The listing builds one solid part. Answer for the finished solid, in the listing's coordinates (mm). Round coordinates to 2 decimals unless told otherwise and drop trailing zeros. Order: outer loops, then holes, each group sorted by start corner. A loop starts at its lowest first (then second) coordinate and runs counter-clockwise, first axis right, second up. Notation, with made-up numbers: (15.25, 56) -> (64.25, 56) arc R20 cw to (64.25, 62) -> close; hole circle Ø10 at (53, 80). An arc over 180 degrees is marked (long way). Answer in a Markdown table with one row per item. Add a question column.
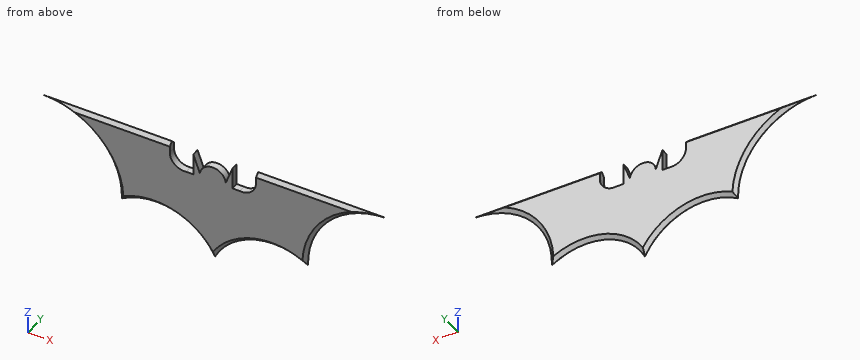
```python
from build123d import *

# Parameters (mm, degrees)
F1_DEPTH = 1.27
F2_SIZE  = 1.26999


# Not quite as in the source:
# - a fillet or chamfer is up to 0.001 mm smaller than in the source, because OpenCascade refuses the exact size
# - a feature names something its author has since deleted; it is built from what else it names


with BuildPart() as f1:
    # F0 (on Front) → F1 (new body, symmetric)
    with BuildSketch(Plane.XZ):
        with BuildLine():
            Line((-15.113, 14.986), (-60.325, 14.986))
            ThreePointArc((-60.325, 14.986), (-40.4178225843, 6.541072822), (-32.6550259817, -13.6418778197))
            ThreePointArc((-32.6550259817, -13.6418778197), (-14.2166113122, -11.1006310534), (0, -23.114))
            ThreePointArc((0, -23.114), (14.2166113122, -11.1006310534), (32.6550259817, -13.6418778197))
            ThreePointArc((32.6550259817, -13.6418778197), (40.4178225843, 6.541072822), (60.325, 14.986))
            Line((60.325, 14.986), (15.113, 14.986))
            Line((15.113, 14.986), (15.113, 11.43))
            ThreePointArc((15.113, 11.43), (13.3972241951, 7.623637489), (9.4089072578, 6.3884815532))
            Line((9.4089072578, 6.3884815532), (6.8689072578, 6.3884815532))
            Line((6.8689072578, 6.3884815532), (6.8689072578, 14.0084815532))
            Line((6.8689072578, 14.0084815532), (4.5436901303, 7.62))
            ThreePointArc((4.5436901303, 7.62), (0, 11.684), (-4.5436901303, 7.62))
            Line((-4.5436901303, 7.62), (-6.8689072578, 14.0084815532))
            Line((-6.8689072578, 14.0084815532), (-6.8689072578, 6.3884815532))
            Line((-6.8689072578, 6.3884815532), (-9.4089072578, 6.3884815532))
            ThreePointArc((-9.4089072578, 6.3884815532), (-13.3972241951, 7.623637489), (-15.113, 11.43))
            Line((-15.113, 11.43), (-15.113, 14.986))
        make_face()
    extrude(amount=F1_DEPTH, both=True)

    # F2 (size 1.27 in the source; OpenCascade refuses exactly that, so slightly less here)
    f2_edges = [f1.edges().sort_by_distance(p)[0] for p in [
        (-40.417823, -1.27, 6.541073),
        (-37.719, -1.27, 14.986),
        (-14.216611, -1.27, -11.100631),
        (-14.216611, 1.27, -11.100631),
        (-40.417823, 1.27, 6.541073),
        (-37.719, 1.27, 14.986),
        (37.719, -1.27, 14.986),
        (40.417823, -1.27, 6.541073),
        (14.216611, -1.27, -11.100631),
        (37.719, 1.27, 14.986),
        (40.417823, 1.27, 6.541073),
        (14.216611, 1.27, -11.100631),
    ]]
    chamfer(f2_edges, length=F2_SIZE)


solid = f1.part
```
1. The part is cut by section A-A (y = -0.65). Give the vertices of the cut face in (x, z) (3 decimals), then the cut area to 3 significant figures.
2. This flat-tipped pin is pushed along its axis until it touches: pin 1 (1.3 mm diameter, centred on y = 0, z = 10.5, fed in from +X). Where does it stop, or does it pass through?
3. Straight lines are drawn through the part: line 1 along X through (y, z) = (-0.6, 9); line 2 along X through (y, z) = (-1, 9); line 3 along Z through (x, y) = (-28, 0). For each, find the intervals that lie inside material, in ascending order.
Report:
| question | item | result |
|---|---|---|
| 1 | outline | (-51.841, 14.336) arc R28.336 cw to (-31.99, -12.497) arc R23.51 cw to (0, -21.699) arc R23.51 cw to (31.99, -12.497) arc R28.336 cw to (51.841, 14.336) -> (15.113, 14.336) -> (15.113, 11.43) arc R5.08 cw to (9.409, 6.388) -> (6.869, 6.388) -> (6.869, 14.008) -> (4.544, 7.62) arc R4.572 ccw to (-4.544, 7.62) -> (-6.869, 14.008) -> (-6.869, 6.388) -> (-9.409, 6.388) arc R5.08 cw to (-15.113, 11.43) -> (-15.113, 14.336) -> close |
| 1 | area | 1,810 mm^2 |
| 2 | pin 1 | stops at x = 46.26 |
| 3 | line 1 | x = -42.18 to -14.49, -6.87 to -5.05, -4.16 to 4.16, 5.05 to 6.87, 14.49 to 42.18 |
| 3 | line 2 | x = -41.56 to -14.49, -6.87 to -5.05, -4.16 to 4.16, 5.05 to 6.87, 14.49 to 41.56 |
| 3 | line 3 | z = -11.43 to 14.99 |
